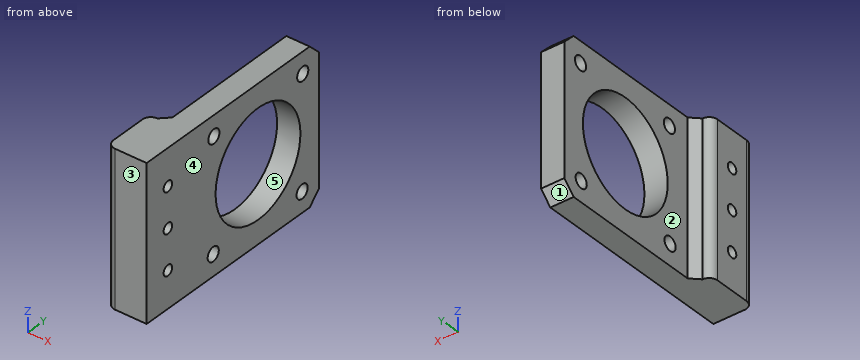
```python
from build123d import *

# Parameters (mm, degrees)
SKETCH1_W                                           = 92.56
SKETCH1_H                                           = 46
BOSS_EXTRUDE1_DEPTH                                 = 6
SKETCH2_W                                           = 7
SKETCH2_H                                           = 46
BOSS_EXTRUDE2_DEPTH                                 = 54
SKETCH3_R                                           = 16
CUT_EXTRUDE1_DEPTH                                  = 120.512985069
SKETCH4_R                                           = 16
CUT_EXTRUDE2_DEPTH                                  = 117.616266447
F_4_2_4_2_DIAMETER_HOLE1_D                          = 4.2
F_4_2_4_2_DIAMETER_HOLE2_D                          = 4.2
CHAMFER1_SIZE                                       = 3.5
CHAMFER2_SIZE                                       = 6
BOSS_EXTRUDE3_DEPTH                                 = 46
FILLET1_R                                           = 2.5
CHAMFER3_SIZE                                       = 2.5
FILLET2_R                                           = 2.5
M3_CLEARANCE_HOLE1_D                                = 3.2
M3_CLEARANCE_HOLE1_DEPTH                            = 30
M3_CLEARANCE_HOLE1_TIP                              = 0.96137699
CSK_FOR_M3_COUNTERSUNK_FLAT_HEAD_SCREW2_D           = 3.6
CSK_FOR_M3_COUNTERSUNK_FLAT_HEAD_SCREW2_DEPTH       = 30
CSK_FOR_M3_COUNTERSUNK_FLAT_HEAD_SCREW2_CSINK_D     = 6.3
CSK_FOR_M3_COUNTERSUNK_FLAT_HEAD_SCREW2_CSINK_ANGLE = 90
CSK_FOR_M3_COUNTERSUNK_FLAT_HEAD_SCREW2_TIP         = 1.081549114
SKETCH18_W                                          = 2.5
SKETCH18_H                                          = 5.65
CUT_EXTRUDE4_DEPTH                                  = 121.623188484


with BuildPart() as part:
    # Sketch1 → Boss-Extrude1 (new body)
    with BuildSketch(Plane(origin=(0, 0, 0), x_dir=(1, 0, 0), z_dir=(0, 1, 0))):
        with Locations((46.28, 23)):
            Rectangle(SKETCH1_W, SKETCH1_H)
    extrude(amount=BOSS_EXTRUDE1_DEPTH)

    # Sketch2 → Boss-Extrude2 (add)
    with BuildSketch(Plane(origin=(0, 6, 0), x_dir=(1, 0, 0), z_dir=(0, 1, 0))):
        with Locations((89.06, 23)):
            Rectangle(SKETCH2_W, SKETCH2_H)
        with Locations((3.5, 23)):
            Rectangle(SKETCH2_W, SKETCH2_H)
    extrude(amount=BOSS_EXTRUDE2_DEPTH)

    # Sketch3 → Cut-Extrude1 (cut, through all)
    with BuildSketch(Plane(origin=(92.56, 0, 0), x_dir=(0, 0, -1), z_dir=(1, 0, 0))):
        with Locations((23, 37)):
            Circle(SKETCH3_R)
    extrude(amount=-CUT_EXTRUDE1_DEPTH, mode=Mode.SUBTRACT)

    # Sketch4 → Cut-Extrude2 (cut, through all)
    with BuildSketch(Plane(origin=(0, 6, 0), x_dir=(1, 0, 0), z_dir=(0, 1, 0))):
        with Locations(Location((46.28, 23, 0), (0, 0, 270))):
            Circle(SKETCH4_R)
    extrude(amount=-CUT_EXTRUDE2_DEPTH, mode=Mode.SUBTRACT)

    # Ø4.2 (4.2) Diameter Hole1 (through all)
    with Locations(Plane(origin=(0, 0, 0), x_dir=(-1, 0, 0), z_dir=(0, -1, 0))):
        with Locations((-63.165621688, 39.642079068), (-29.637920932, 39.885621688), (-29.394378312, 6.357920932), (-62.922079068, 6.114378312)):
            Hole(F_4_2_4_2_DIAMETER_HOLE1_D / 2)

    # Ø4.2 (4.2) Diameter Hole2 (through all)
    with Locations(Plane.ZY):
        with Locations((-39.885621688, 53.642079068), (-6.357920932, 53.885621688), (-6.114378312, 20.357920932), (-39.642079068, 20.114378312)):
            Hole(F_4_2_4_2_DIAMETER_HOLE2_D / 2)

    # Chamfer1
    chamfer1_edges = [part.edges().sort_by_distance(p)[0] for p in [
        (89.06, 60, -46),
        (89.06, 60, 0),
        (3.5, 60, 0),
        (3.5, 60, -46),
    ]]
    chamfer(chamfer1_edges, length=CHAMFER1_SIZE)

    # Chamfer2
    chamfer2_edges = [part.edges().sort_by_distance(p)[0] for p in [
        (85.56, 6, -23),
        (7, 6, -23),
    ]]
    chamfer(chamfer2_edges, length=CHAMFER2_SIZE)

    # Sketch10 → Boss-Extrude3 (add)
    with BuildSketch(Plane(origin=(0, 0, -46), x_dir=(-1, 0, 0), z_dir=(0, 0, -1))):
        Polygon((0, 11), (5, 11), (5, -5), (-11, -5), (-11, 0), (0, 0), align=None)
        Polygon((-81.56, 0), (-92.56, 0), (-92.56, 11), (-97.56, 11), (-97.56, -5), (-81.56, -5), align=None)
    extrude(amount=-BOSS_EXTRUDE3_DEPTH)

    # Fillet1
    fillet1_edges = [part.edges().sort_by_distance(p)[0] for p in [
        (-5, 11, -23),
        (11, -5, -23),
        (81.56, -5, -23),
        (97.56, 11, -23),
    ]]
    fillet(fillet1_edges, radius=FILLET1_R)

    # Chamfer3
    chamfer3_edges = [part.edges().sort_by_distance(p)[0] for p in [
        (92.56, 11, -23),
        (81.56, 0, -23),
        (11, 0, -23),
        (0, 11, -23),
    ]]
    chamfer(chamfer3_edges, length=CHAMFER3_SIZE - 0.0001)  # a hair under: the kernel refuses the full size

    # Fillet2
    fillet2_edges = [part.edges().sort_by_distance(p)[0] for p in [
        (-5, -5, -23),
        (97.56, -5, -23),
    ]]
    fillet(fillet2_edges, radius=FILLET2_R)

    # M3 Clearance Hole1
    with Locations(Plane.ZY.offset(5)):
        with Locations((-11, 3), (-23, 3), (-35, 3)):
            Hole(M3_CLEARANCE_HOLE1_D / 2, depth=M3_CLEARANCE_HOLE1_DEPTH)
            with Locations((0, 0, -(M3_CLEARANCE_HOLE1_DEPTH + M3_CLEARANCE_HOLE1_TIP / 2))):  # 118° drill point
                Cone(0, M3_CLEARANCE_HOLE1_D / 2, M3_CLEARANCE_HOLE1_TIP, mode=Mode.SUBTRACT)

    # CSK for M3 Countersunk Flat Head Screw2
    with Locations(Plane(origin=(97.56, 0, 0), x_dir=(0, 0, -1), z_dir=(1, 0, 0))):
        with Locations((11, 3), (23, 3), (35, 3)):
            CounterSinkHole(CSK_FOR_M3_COUNTERSUNK_FLAT_HEAD_SCREW2_D / 2, CSK_FOR_M3_COUNTERSUNK_FLAT_HEAD_SCREW2_CSINK_D / 2, depth=CSK_FOR_M3_COUNTERSUNK_FLAT_HEAD_SCREW2_DEPTH, counter_sink_angle=CSK_FOR_M3_COUNTERSUNK_FLAT_HEAD_SCREW2_CSINK_ANGLE)
            with Locations((0, 0, -(CSK_FOR_M3_COUNTERSUNK_FLAT_HEAD_SCREW2_DEPTH + CSK_FOR_M3_COUNTERSUNK_FLAT_HEAD_SCREW2_TIP / 2))):  # 118° drill point
                Cone(0, CSK_FOR_M3_COUNTERSUNK_FLAT_HEAD_SCREW2_D / 2, CSK_FOR_M3_COUNTERSUNK_FLAT_HEAD_SCREW2_TIP, mode=Mode.SUBTRACT)

    # Sketch18 → Cut-Extrude4 (cut, through all)
    with BuildSketch(Plane(origin=(0, 6, 0), x_dir=(1, 0, 0), z_dir=(0, 1, 0))):
        with Locations((22, 23)):
            Rectangle(SKETCH18_W, SKETCH18_H)
        with Locations((22, 35)):
            Rectangle(SKETCH18_W, SKETCH18_H)
        with Locations((22, 11)):
            Rectangle(SKETCH18_W, SKETCH18_H)
    cut_extrude4 = extrude(amount=-CUT_EXTRUDE4_DEPTH, mode=Mode.SUBTRACT)

    # Mirror1: Cut-Extrude4 across plane
    add(cut_extrude4.mirror(Plane.ZY.offset(-46.28)), mode=Mode.SUBTRACT)

    # SurfaceCut3
    split(bisect_by=Plane(origin=(7, 0, 0), x_dir=(0, 0, -1), z_dir=(1, 0, 0)), keep=Keep.BOTTOM)


solid = part.part
```
The listing builds one solid part. Answer for the finished solid, in the listing's coordinates (mm). Face numbers are marked on the shaded views. A direction names the side the tool comes from. Round coordinates to 2 decimals unless told otherwise and drop trailing zeros. Loops run counter-clockwise (first coordinate to the right, second up) from the corner with the lowest first, then second, coordinate; pieces in that order, holes last. Notation, with made-up numbers: (31.5, 24) - (51.5, 24) arc R19 ccw to (51.5, 45) - close; hole circle Ø3 at (70.5, 4). An arc over 180 degrees is marked (long way). Use one line per item in the form item = value. Start each with the question number.
1. Given pin 1 Ø1.5 at (x, z) = (-3.5, -31.5) entering from -Y; pin 2 Ø6.5 at (y, z) = (53.89, -6.36) entering from -X, each flat-ended and moving along its own axis, determine where each tip first touches the part or whether it passes through.
2. Consider line 1 (Y direction, x = 0.25, z = -34); line 2 (X direction, y = 25, z = -9.5); line 3 (Y direction, x = -2.75, z = -32). Determine where each line is inside the solid, lowest interval first. Write a range as [from, to].
3. A tool of negligible diameter and unlimited length cuts with its end or side. For the marked faces 1 and 2, from which of +Z, -Z, +X, -X, +Y, -Y can it reach the whole face along a straight path? Write none if from no direction.
4. For a pull along Y with two mould halves and no side action, classify the marked faces 3, 4 and 5 as pulls with the +Y half, pulls with the -Y half, needs draft (parallel to the pull), parting line crosses it, or undercut.
5. The part is cut by section B-B on z = -23. Give the number of separate pieces and of enclosed holes in the cut face, then the cut area to 3 significant figures.
6. The part is cut by section D-D on x = -3.5. Determine the outline of the cut face in (y, z).
7. The part is cut by section C-C on y = 3. Determine the outline of the cut face in (x, z), then the cut area to 3 significant figures.
8. The part is cut by section A-A on y = 37. Determine the outline of the cut face in (x, z).
Geometry check:
q1.pin_1 = -4.99
q1.pin_2 = 0
q2.line_1 = [-5, 1.75], [4.25, 25.38], [48.62, 60]
q2.line_2 = [0, 7]
q2.line_3 = [-4.99, 10.99]
q3.face_1 = -Z, +X, -X, +Y
q3.face_2 = +Z, -Z, -X, +Y
q4.face_3 = pulls with the -Y half
q4.face_4 = needs draft
q4.face_5 = undercut
q5.separate_pieces = 3
q5.enclosed_holes = 0
q5.area = 273 mm^2
q6.outline = (-4.79, -46) - (10.79, -46) - (10.79, 0) - (-4.79, 0) - close; hole circle Ø3.2 at (3, -35); hole circle Ø3.2 at (3, -23); hole circle Ø3.2 at (3, -11)
q7.outline = (-5, -46) - (7, -46) - (7, -36.6) - (-5, -36.6) - close; (-5, -33.4) - (7, -33.4) - (7, -24.6) - (-5, -24.6) - close; (-5, -21.4) - (7, -21.4) - (7, -12.6) - (-5, -12.6) - close; (-5, -9.4) - (7, -9.4) - (7, 0) - (-5, 0) - close
q7.area = 437 mm^2
q8.outline = (0, -46) - (7, -46) - (7, -39) - (0, -39) - close; (0, -7) - (7, -7) - (7, 0) - (0, 0) - close
